Autodesk Inventor part; units mm, degrees
ref_plane "YZ Plane" through (0, 0, 0) normal (1, 0, 0) x (0, 1, 0)
ref_plane "XZ Plane" through (0, 0, 0) normal (0, 1, 0) x (-1, 0, 0)
ref_plane "XY Plane" through (0, 0, 0) normal (0, 0, 1) x (1, 0, 0)
sketch "Sketch1" plane through (0, 0, 0) normal (0, 1, 0) x (-1, 0, 0)
  circle A0 centre (0, 0) radius 5
  dimension "d3" = 10
extrude "Extrusion1" add sketch "Sketch1" along normal mid plane 10
sketch "Sketch2" plane through (0, 5, 0) normal (0, 1, 0) x (1, 0, 0)
  line L0 (1.2772, 2.5889) -> (2.8806, 0.1884)
  line L1 (2.8806, 0.1884) -> (1.6034, -2.4005)
  line L2 (1.6034, -2.4005) -> (-1.2772, -2.5889)
  line L3 (-1.2772, -2.5889) -> (-2.8806, -0.1884)
  line L4 (-2.8806, -0.1884) -> (-1.6034, 2.4005)
  line L5 (-1.6034, 2.4005) -> (1.2772, 2.5889)
  point P0 (0, 0)
  point P1 (0, 0)
  dimension "d2" = 5
extrude "Extrusion2" cut sketch "Sketch2" against normal blind 5.5
thread "Thread1"
chamfer "Chamfer1" distance 0.5 angle 45 2 edges at (5, 5, 0) (5, -5, 0)
properties part number "M10_HEX"
Verification items for the finished model (mm, model axes). A direction names the side the tool comes from. Give positions to 0.01 mm unless a question says otherwise; leave off trailing zeros. Write each loop counter-clockwise with the first axis right and the second up, starting at its lowest first coordinate (ties: lowest second). Pieces come first, ordered by that corner, then holes.
(1) Mould release check, pull along X, two halves, no side actions. Record for faces 3 (the face through (2.25, 2.29, 1.09)), 4 (the face through (-2, 5, -2)), 5 (the face through (-2.068, 2.288, 1.405)), 6 (the face through (1.08, -0.06, 4.88)): +X half, -X half, draft (parallel to the pull), parting line (faces both ways), or undercut.
(2) Access from +Z, -Z, +X, -X, +Y, -Y to the whole of each face (thin tool, end or side, straight path). Record for faces 1 (the face through (0, -0.5, 0)), 2 (the face through (0, -5, 0)).
(3) Material ranges on line 1 (Z direction, x = 0.5, y = 2.5); line 2 (Z direction, x = 1.5, y = 4.75); line 3 (Y direction, x = 0.5, z = -2.25), recorded low to high.
(4) Cross-section at D-D (z = 0). Enter the section's corners in (x, y), plus the area to 3 significant figures.
(5) Gauge pin test, flat ends, axial feed: pin 1 (3 mm diameter, centred on x = -2, y = 3, fed in from -Z); pin 2 (3 mm diameter, centred on y = -3, z = -3.5, fed in from -X); pin 3 (4 mm diameter, centred on x = 3.5, y = 0.5, fed in from -Z). Record the tip position at first contact, or that the pin passes through.
(6) Cross-section at C-C (x = 0). Enter the section's corners in (y, z).
(7) Cross-section at A-A (y = 1). Enter the section's corners in (x, z).
(8) Cross-section at B-B (y = -3.75). Enter the section's corners in (x, z).
Worked out:
1. face 3: undercut
1. face 4: draft
1. face 5: undercut
1. face 6: parting line
2. face 1: +Y
2. face 2: +Z, -Z, +X, -X, -Y
3. line 1: z = -4.97 to -2.54, 2.47 to 4.97
3. line 2: z = -4.51 to -2.26, 2.41 to 4.51
3. line 3: y = -5 to -0.5
4. outline: (-5, -4.5) - (-4.5, -5) - (4.5, -5) - (5, -4.5) - (5, 4.5) - (4.5, 5) - (2.79, 5) - (2.79, -0.5) - (-2.79, -0.5) - (-2.79, 5) - (-4.5, 5) - (-5, 4.5) - close
4. area: 68.8 mm2
5. pin 1: stops at z = -4.97
5. pin 2: stops at x = -4.58
5. pin 3: stops at z = -4.77
6. outline: (-5, -4.5) - (-4.5, -5) - (4.5, -5) - (5, -4.5) - (5, -2.51) - (-0.5, -2.51) - (-0.5, 2.51) - (5, 2.51) - (5, 4.5) - (4.5, 5) - (-4.5, 5) - (-5, 4.5) - close
7. outline: circle Ø10 at (0, 0); hole (-2.88, 0.19) - (-1.6, -2.4) - (1.28, -2.59) - (2.88, -0.19) - (1.6, 2.4) - (-1.28, 2.59) - close
8. outline: circle Ø10 at (0, 0)
